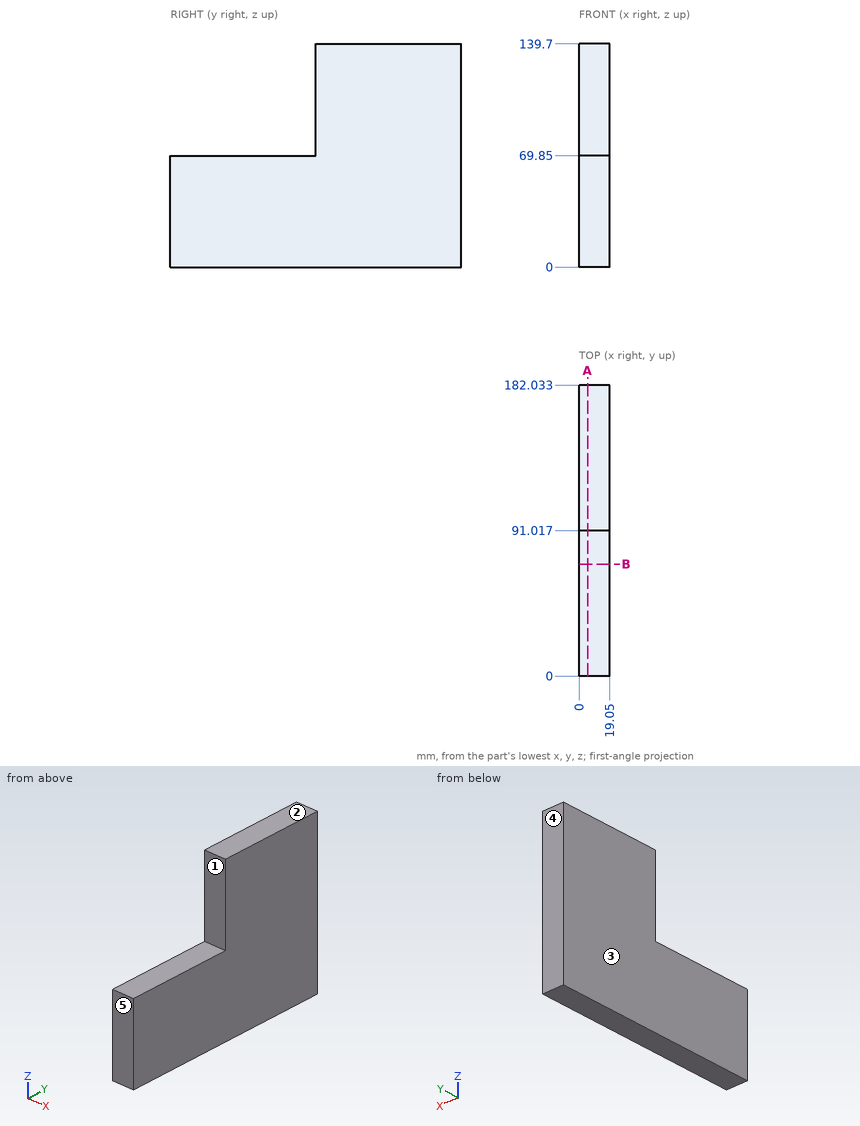
Drawing for the job (mm, zero at the part's lowest x, y, z). A direction names the side the tool comes from. Round coordinates to 2 decimals unless told otherwise and drop trailing zeros. Loops run counter-clockwise (first coordinate to the right, second up) from the corner with the lowest first, then second, coordinate; pieces in that order, holes last.
1. Tool access for the marked faces 1 and 2: list every direction of +Z, -Z, +X, -X, +Y, -Y with a clear straight run to the whole face (end or side of a thin tool).
Check values:
face 1: +Z, +X, -X, -Y
face 2: +Z, +X, -X, +Y, -Y
2. Wall check: probe 1 along Z at (x, y) = (13.5, 63.5); probe 2 along Y at (x, z) = (2.5, 98.5). Give the ranges that are in metal, low to high.
Check values:
probe 1: z = 0 to 69.85
probe 2: y = 91.02 to 182.03
3. Band-saw the part on B-B, the plane y = 70. List the corners of the cut face in (x, z), and give its area (3 significant figures).
Check values:
outline: (0, 0) - (19.05, 0) - (19.05, 69.85) - (0, 69.85) - close
area: 1,330 mm2
4. Mould opens along Y. For the marked faces 3, 4 and 5 say: +Y half, -Y half, draft (parallel to the pull), parting line (faces both ways), or undercut.
Check values:
face 3: draft
face 4: +Y half
face 5: -Y half
5. Band-saw the part on A-A, the plane x = 5.25. List the corners of the cut face in (y, z).
Check values:
outline: (0, 0) - (182.03, 0) - (182.03, 139.7) - (91.02, 139.7) - (91.02, 69.85) - (0, 69.85) - close
6. Drop flat-ended pins along their axis: P1, Ø8, axis at x = 17, y = 140, coming from the -Z side; P2, Ø5.5, axis at x = 7, y = 53.5, coming from the +Z side. Give the stop position or say it passes through.
Check values:
P1: stops at z = 0
P2: stops at z = 69.85
